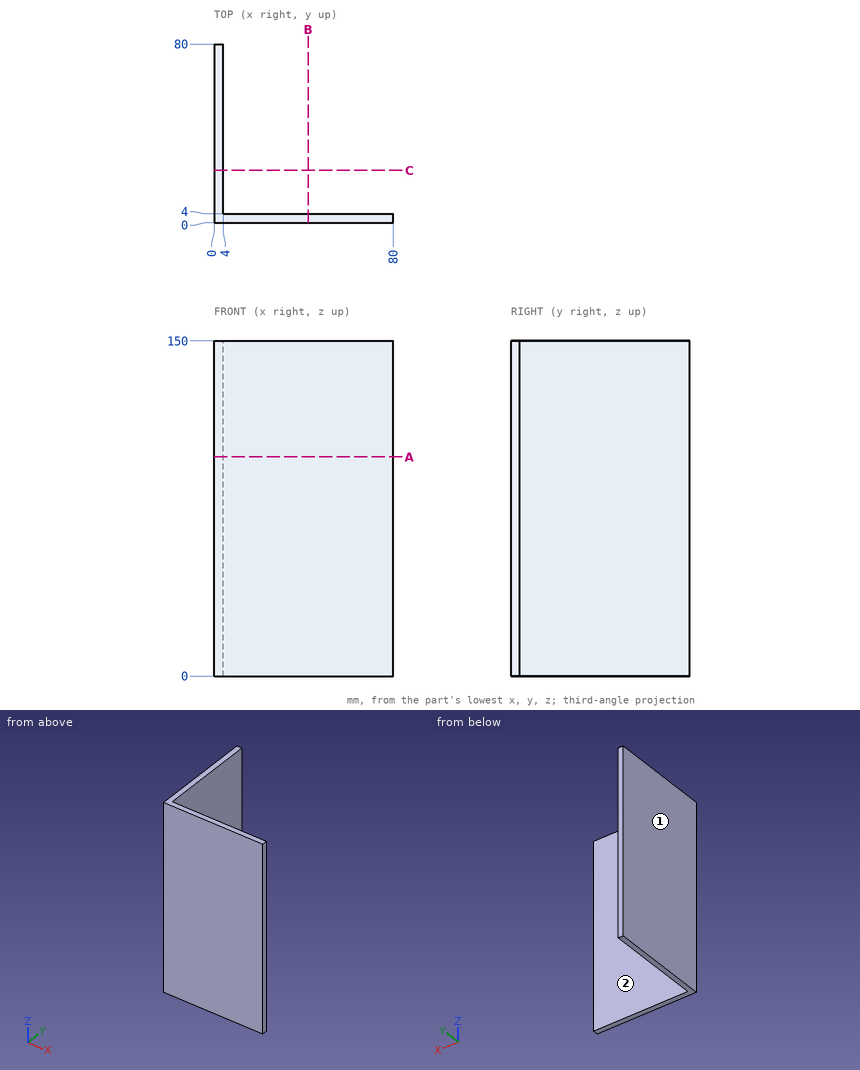
For this review, use the dimensioned drawing (mm, ordinates from the lowest corner) and the shaded views. A direction names the side the tool comes from. Coordinates: 2 decimals unless noted, no trailing zeros. Loops run counter-clockwise (first coordinate to the right, second up) from the corner with the lowest first, then second, coordinate; pieces in that order, holes last. Notation, with made-up numbers: (18, -25.75) -> (33, -25.75) arc R14 ccw to (33, -3.75) -> close; hole circle Ø3 at (76, 30). An arc over 180 degrees is marked (long way). Use a Markdown table: item, result. Add a question column.
1. Add section A-A on z = 98. Write out the cut boundary in (x, y), plus the area to 3 significant figures.
2. To check wall thickness, follow line 1 (X direction, y = 50.5, z = 71.5). State the ranges of the line that lie inside material, in increasing order.
3. Machinability: for the marked faces 1 and 2, which of the approach directions +Z, -Z, +X, -X, +Y, -Y give a long, thin tool a straight path to every point of the face, cutting with its end or side? Answer none if there is none.
4. Add section B-B on x = 42. Write out the cut boundary in (y, z).
5. Clearance check with flat-ended pins moving along their axes: pin 1 Ø1 at (y, z) = (52, 18.5) entering from +X; pin 2 Ø6 at (y, z) = (24, 51) entering from -X. State where each tip first meets the part, or that it passes through.
Returned:
| question | item | result |
|---|---|---|
| 1 | outline | (0, 0) -> (80, 0) -> (80, 4) -> (4, 4) -> (4, 80) -> (0, 80) -> close |
| 1 | area | 624 mm² |
| 2 | line 1 | x = 0 to 4 |
| 3 | face 1 | +Z, -Z, -X, +Y, -Y |
| 3 | face 2 | +Z, -Z, +X, +Y |
| 4 | outline | (0, 0) -> (4, 0) -> (4, 150) -> (0, 150) -> close |
| 5 | pin 1 | stops at x = 4 |
| 5 | pin 2 | stops at x = 0 |
